Source: three-view drawing plus pictorial views. Frame: mm from the lowest corner of the part. Give positions to 0.01 mm unless a question says otherwise; leave off trailing zeros. Loops run counter-clockwise (first coordinate to the right, second up) from the corner with the lowest first, then second, coordinate; pieces in that order, holes last. Notation, with made-up numbers: (89, 7) - (139, 7) arc R21 ccw to (139, 13) - close; hole circle Ø2 at (66.5, -8.75). An arc over 180 degrees is marked (long way). Answer in a Markdown table with one row per item.
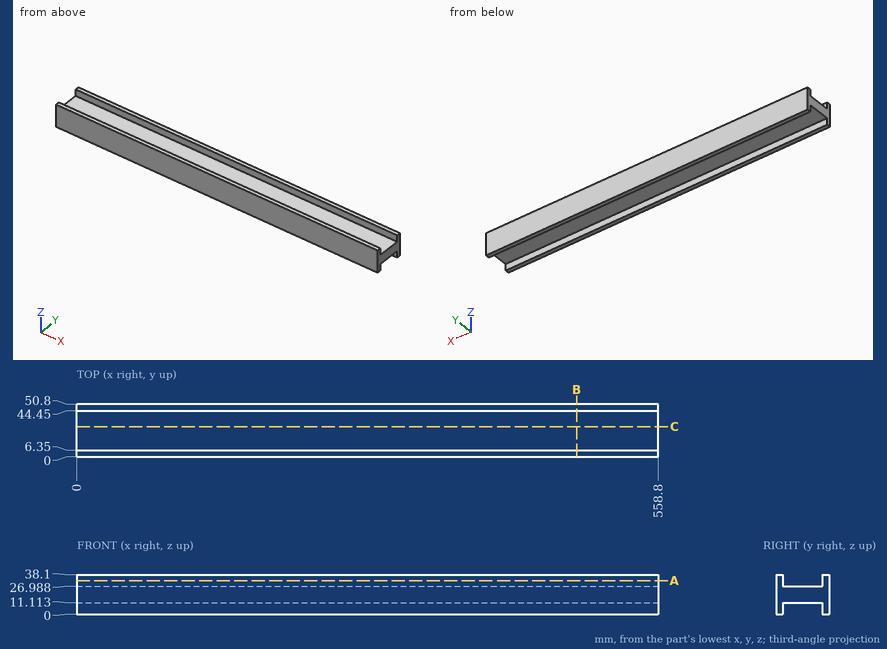
Q1. Cut plane B-B (x = 480.5). Output: boundary loops of the cut face in (y, z), and give its area (3 significant figures).
Check values:
| item | result |
|---|---|
| outline | (0, 0) - (6.35, 0) - (6.35, 11.11) - (44.45, 11.11) - (44.45, 0) - (50.8, 0) - (50.8, 38.1) - (44.45, 38.1) - (44.45, 26.99) - (6.35, 26.99) - (6.35, 38.1) - (0, 38.1) - close |
| area | 1,090 mm² |
Q2. Material intervals for line 1 along Y through (x, z) = (444.5, 28.5); line 2 along Z through (x, y) = (107, 18.5), sorted ascending.
Check values:
| item | result |
|---|---|
| line 1 | 0 to 6.35, 44.45 to 50.8 |
| line 2 | 11.11 to 26.99 |
Q3. Cut plane A-A (z = 32.5). Output: boundary loops of the cut face in (x, y).
Check values:
| item | result |
|---|---|
| outline | (0, 0) - (558.8, 0) - (558.8, 6.35) - (0, 6.35) - close; (0, 44.45) - (558.8, 44.45) - (558.8, 50.8) - (0, 50.8) - close |
Q4. Cut plane C-C (y = 29). Output: boundary loops of the cut face in (x, z).
Check values:
| item | result |
|---|---|
| outline | (0, 11.11) - (558.8, 11.11) - (558.8, 26.99) - (0, 26.99) - close |
Q5. First-contact query: pin 1 (11.5 mm diameter, centred on x = 249, y = 22.5, fed in from -Z); pin 2 (2 mm diameter, centred on x = 358.5, y = 22.5, fed in from +Z); pin 3 (2 mm diameter, centred on x = 69, z = 22.5, fed in from -Y). Flat tips, straight axial feed; report the tip coordinate or a pass-through.
Check values:
| item | result |
|---|---|
| pin 1 | z = 11.11 |
| pin 2 | z = 26.99 |
| pin 3 | y = 0 |
